from build123d import *

# Parameters (mm, degrees)
SKETCH_1_R               = 6.45
EXTRUDE_1_DEPTH          = 15
SKETCH_2_W               = 29.5
SKETCH_2_H               = 18
EXTRUDE_2_DEPTH          = 3
EXTRUDE_START            = 14.75
SKETCH_3_R               = 1.65
EXTRUDE_3_DEPTH          = 5
EXTRUDE_START_2          = -14.75
SKETCH_3_2_R             = 1.65
EXTRUDE_4_DEPTH          = 5
EXTRUDE_5_DEPTH          = 10
FILLET_1_R               = 5
SKETCH_5_R               = 2.5
CUT_EXTRUDE_1_DEPTH      = 19
CHAMFER_1_SIZE           = 1
CHAMFER_2_SIZE           = 1
CUT_EXTRUDE_2_DEPTH      = 15.75
CUT_EXTRUDE_2_DEPTH_BACK = 15.75
FILLET_2_R               = 1


with BuildPart() as part:
    # ｽｹｯﾁ1 → ﾎﾞｽ - 押し出し1 (new body)
    with BuildSketch(Plane.XY):
        Circle(SKETCH_1_R)
    extrude(amount=EXTRUDE_1_DEPTH)

    # ｽｹｯﾁ2 → ﾎﾞｽ - 押し出し2 (add)
    with BuildSketch(Plane.XY.offset(15)):
        Rectangle(SKETCH_2_W, SKETCH_2_H)
    extrude(amount=EXTRUDE_2_DEPTH)

    # ｽｹｯﾁ3 → ﾎﾞｽ - 押し出し3 (add)
    with BuildSketch(Plane(origin=(0, 0, 0), x_dir=(0, 0, -1), z_dir=(1, 0, 0)).offset(EXTRUDE_START)):
        with BuildLine():
            Line((-18, 9), (-31.333333333, 13.714045208))
            ThreePointArc((-31.333333333, 13.714045208), (-37.386897866, 11.398984601), (-36.069570429, 5.053135753))
            Line((-36.069570429, 5.053135753), (-18, -9))
            Line((-18, -9), (-18, 9))
        make_face()
        with Locations((-33, 9)):
            Circle(SKETCH_3_R, mode=Mode.SUBTRACT)
    extrude(amount=-EXTRUDE_3_DEPTH)

    # ｽｹｯﾁ3<2> → ﾎﾞｽ - 押し出し4 (add)
    with BuildSketch(Plane(origin=(0, 0, 0), x_dir=(0, 0, -1), z_dir=(1, 0, 0)).offset(EXTRUDE_START_2)):
        with BuildLine():
            Line((-18, 9), (-31.333333333, 13.714045208))
            ThreePointArc((-31.333333333, 13.714045208), (-37.386897866, 11.398984601), (-36.069570429, 5.053135753))
            Line((-36.069570429, 5.053135753), (-18, -9))
            Line((-18, -9), (-18, 9))
        make_face()
        with Locations((-33, 9)):
            Circle(SKETCH_3_2_R, mode=Mode.SUBTRACT)
    extrude(amount=EXTRUDE_4_DEPTH)

    # ｽｹｯﾁ4 → ﾎﾞｽ - 押し出し5 (add)
    with BuildSketch(Plane.XZ.offset(9)):
        Polygon((-14.75, 15), (14.75, 15), (14.75, 18), (9.75, 18), (-9.75, 18), (-14.75, 18), align=None)
    extrude(amount=EXTRUDE_5_DEPTH)

    # ﾌｨﾚｯﾄ1
    fillet_1_edges = [part.edges().sort_by_distance(p)[0] for p in [
        (-14.75, -19, 16.5),
        (14.75, -19, 16.5),
    ]]
    fillet(fillet_1_edges, radius=FILLET_1_R)

    # ｽｹｯﾁ5 → ｶｯﾄ - 押し出し1 (cut, through all)
    with BuildSketch(Plane.XY.offset(18)):
        with Locations((0, -14)):
            Circle(SKETCH_5_R)
        with Locations((-9.75, -14)):
            Circle(SKETCH_5_R)
        with Locations((9.75, -14)):
            Circle(SKETCH_5_R)
    extrude(amount=-CUT_EXTRUDE_1_DEPTH, mode=Mode.SUBTRACT)

    # 面取り1
    chamfer_1_edges = [part.edges().sort_by_distance(p)[0] for p in [
        (7.25, -14, 15),
        (7.25, -14, 18),
        (-12.25, -14, 15),
        (-12.25, -14, 18),
        (-2.5, -14, 15),
        (-2.5, -14, 18),
    ]]
    chamfer(chamfer_1_edges, length=CHAMFER_1_SIZE)

    # 面取り2
    chamfer_2_edges = [part.edges().sort_by_distance(p)[0] for p in [
        (-14.75, 9, 16.5),
        (0, 9, 15),
        (14.75, 9, 16.5),
        (-14.75, 11.357022604, 24.666666667),
        (-14.75, 11.398984601, 37.386897866),
        (-14.75, -1.973432123, 27.034785215),
        (14.75, 11.357022604, 24.666666667),
        (14.75, 11.398984601, 37.386897866),
        (14.75, -1.973432123, 27.034785215),
    ]]
    chamfer(chamfer_2_edges, length=CHAMFER_2_SIZE)

    # ｽｹｯﾁ6 → ｶｯﾄ - 押し出し2 (cut, two sides)
    with BuildSketch(Plane(origin=(0, 0, 0), x_dir=(0, 0, -1), z_dir=(1, 0, 0))) as cut_extrude_2_sk:
        with BuildLine():
            Line((-8.928941916, -0.825), (-9.405255888, 0))
            Line((-9.405255888, 0), (-8.928941916, 0.825))
            ThreePointArc((-8.928941916, 0.825), (-5.85, 0), (-8.928941916, -0.825))
        make_face()
    extrude(amount=CUT_EXTRUDE_2_DEPTH, mode=Mode.SUBTRACT)
    extrude(cut_extrude_2_sk.sketch, amount=-CUT_EXTRUDE_2_DEPTH_BACK, mode=Mode.SUBTRACT)

    # ﾌｨﾚｯﾄ2
    fillet_2_edges = [part.edges().sort_by_distance(p)[0] for p in [
        (-6.45, 0, 0),
    ]]
    fillet(fillet_2_edges, radius=FILLET_2_R)


solid = part.part
Input: part model. Units: mm. Frame: model coordinates. A direction names the side the tool comes from. Coordinates: 2 decimals unless noted, no trailing zeros. Loops run counter-clockwise (first coordinate to the right, second up) from the corner with the lowest first, then second, coordinate; pieces in that order, holes last.
Q1. Cut plane D-D (y = -15.5). Give the number of separate pieces and of enclosed holes in the cut face, then the cut area to 3 significant figures.
Q2. Set-up query: faces 1 (the face through (9.75, 5, 26)), 2 (the face through (14.75, 3, 23)). Return all of +Z, -Z, +X, -X, +Y, -Y with unobstructed straight access to the full face (end or side cutting, diameter ignored); none if empty.
Q3. Contact query for flat-ended pins moving along their axis: pin 1 (6 mm diameter, centred on x = 11, y = 8, fed in from -Z); pin 2 (8 mm diameter, centred on x = -9.5, z = 4.5, fed in from +Y); pin 3 (1.6 mm diameter, centred on x = 4, z = 16.5, fed in from +Y); pin 4 (4.5 mm diameter, centred on x = -9.75, y = -14, fed in from -Z). Output: stop coordinate, or through.
Q4. Draft query along X for faces 3 (the face through (14.26, 8.49, 16.92)), 4 (the face through (5.96, -2.47, 7.9)), 5 (the face through (0, -5, 18)). Return one class per face: +X half, -X half, draft (parallel to the pull), parting line (faces both ways), or undercut.
Q5. Material intervals for line 1 (X direction, y = -13, z = 16.5); line 2 (Y direction, x = 9.75, z = 16.75); line 3 (Z direction, x = 0, y = 0), sorted ascending.
Q6. Cut plane C-C (z = 33). Output: boundary loops of the cut face in (x, y).
Q7. Cut plane A-A (x = 0). Output: boundary loops of the cut face in (y, z) (3 decimals).
Q8. Cut plane B-B (z = 25.5). Output: boundary loops of the cut face in (x, y).
Working result:
1. separate pieces: 4
1. enclosed holes: 0
1. area: 44.0 mm2
2. face 1: +Z, +Y, -Y
2. face 2: +Z, -Z, +X, +Y, -Y
3. pin 1: stops at z = 15
3. pin 2: stops at y = 3.37
3. pin 3: stops at y = 9
3. pin 4: passes through
4. face 3: +X half
4. face 4: parting line
4. face 5: undercut
5. line 1: x = -14.75 to -12.04, -7.46 to -2.29, 2.29 to 7.46, 12.04 to 14.75
5. line 2: y = -19 to -16.5, -11.5 to 9
5. line 3: z = 0 to 5.85, 9.41 to 18
6. outline: (-14.75, 3.93) - (-13.75, 2.67) - (-9.75, 2.67) - (-9.75, 7.35) - (-14.75, 7.35) - close; (-14.75, 10.65) - (-9.75, 10.65) - (-9.75, 14) - (-13.75, 14) - (-14.75, 13) - close; (9.75, 2.67) - (13.75, 2.67) - (14.75, 3.93) - (14.75, 7.35) - (9.75, 7.35) - close; (9.75, 10.65) - (14.75, 10.65) - (14.75, 13) - (13.75, 14) - (9.75, 14) - close
7. outline: (-19, 15) - (-17.5, 15) - (-16.5, 16) - (-16.5, 17) - (-17.5, 18) - (-19, 18) - close; (-11.5, 16) - (-10.5, 15) - (-6.45, 15) - (-6.45, 1) arc R1 ccw to (-5.45, 0) - (5.45, 0) arc R1 ccw to (6.45, 1) - (6.45, 15) - (8, 15) - (9, 16) - (9, 18) - (-10.5, 18) - (-11.5, 17) - close; hole (-0.825, 8.929) arc R1.65 ccw (long way) to (0.825, 8.929) - (0, 9.405) - close
8. outline: (-14.75, -1.9) - (-13.75, -3.17) - (-9.75, -3.17) - (-9.75, 11.65) - (-13.75, 11.65) - (-14.75, 10.59) - close; (9.75, -3.17) - (13.75, -3.17) - (14.75, -1.9) - (14.75, 10.59) - (13.75, 11.65) - (9.75, 11.65) - close
